Input: part model. Units: mm. Frame: model coordinates. A direction names the side the tool comes from. Round coordinates to 2 decimals unless told otherwise and drop trailing zeros. Loops run counter-clockwise (first coordinate to the right, second up) from the corner with the lowest first, then second, coordinate; pieces in that order, holes last. Notation, with made-up numbers: M 5,68.5 L 54,68.5 A9 cw 54,78.5 Z; hole C 29.5,20 d3. An arc over 180 degrees is marked long. Return JSON: item names as keys, results as strings. Group by question number.
1) Section A-A (y = 0). Output: boundary loops of the cut face in (x, z), plus the area to 3 significant figures.
2) Section C-C (x = 18). Output: boundary loops of the cut face in (y, z), plus the area to 3 significant figures.
3) Section B-B (z = 1.75). Output: boundary loops of the cut face in (x, y), plus the area to 3 significant figures.
4) Section D-D (x = -32). Output: boundary loops of the cut face in (y, z), plus the area to 3 significant figures.
5) Material intervals for line 1 (Z direction, x = -37, y = -14.5); line 2 (Y direction, x = -8, z = 7.25); line 3 (X direction, y = -2.5, z = 22.75), sorted ascending. Write a range as from..to.
6) Contact query for flat-ended pins moving along their axis: P1, Ø5, axis at x = -15, y = -11, coming from the +Z side; P2, Ø10, axis at x = -31.5, z = 13, coming from the -Y side; P3, Ø8.5, axis at x = -24, z = 7, coming from the +Y side. Output: stop coordinate, or through.
7) Access query for faces 4 (the face through (-28, 16.883, 5)), 5 (the face through (-29, 4, 10.668)), 6 (the face through (-20, -2.902, 13)). Directions: +Z, -Z, +X, -X, +Y, -Y. A direction counts if a zero-diameter tool reaches every point of the face in a straight line with its end or side. Return the directions, or none.
8) Mould query, pull axis Y, two halves, no side actions, for faces 1 (the face through (-55.367, 0, 5)), 2 (the face through (8.39, -9.46, 12.52)), 3 (the face through (-29, -16.883, 5)). Classes: +Y half, -Y half, draft (parallel to the pull), parting line (faces both ways), or undercut.
from build123d import *

# Parameters (mm, degrees)
F1_DEPTH = 10.668
F0_R     = 9.6911240881
F2_DEPTH = 25.4
F4_DEPTH = 9.144
F6_DEPTH = 23.4226514116


with BuildPart() as f1:
    # F0 (on Top) → F1 (new body)
    with BuildSketch(Plane.XY):
        with BuildLine():
            ThreePointArc((-1.1775513103, -16.8828442693), (-10.0338594761, 0), (-1.1775513103, 16.8828442693))
            Line((-1.1775513103, 16.8828442693), (-55.3673403338, 16.8828442693))
            Line((-55.3673403338, 16.8828442693), (-55.3673403338, -16.8828442693))
            Line((-55.3673403338, -16.8828442693), (-1.1775513103, -16.8828442693))
        make_face()
    extrude(amount=F1_DEPTH)

    # F0 (on Top) → F2 (join)
    with BuildSketch(Plane.XY):
        with BuildLine():
            ThreePointArc((31.0063367483, 0), (20.0186127494, 18.1716336717), (-1.1775513103, 16.8828442693))
            ThreePointArc((-1.1775513103, 16.8828442693), (-10.0338594761, 0), (-1.1775513103, -16.8828442693))
            ThreePointArc((-1.1775513103, -16.8828442693), (20.0186127494, -18.1716336717), (31.0063367483, 0))
        make_face()
        with Locations((10.4862386361, 0)):
            Circle(F0_R, mode=Mode.SUBTRACT)
    extrude(amount=F2_DEPTH)

    # F3 (on face) → F4 (join)
    with BuildSketch(Plane.XY.offset(10.668)):
        with BuildLine():
            ThreePointArc((-9.8276830676, -2.9015532994), (-10.0338594761, 0), (-9.8276830676, 2.9015532994))
            Line((-9.8276830676, 2.9015532994), (-46.7980072435, 2.9015532994))
            Line((-46.7980072435, 2.9015532994), (-46.7980072435, -2.9015532994))
            Line((-46.7980072435, -2.9015532994), (-9.8276830676, -2.9015532994))
        make_face()
    extrude(amount=F4_DEPTH)

    # F5 (on face) → F6 (cut, through all)
    with BuildSketch(Plane.XZ.offset(2.9015532994)):
        Polygon((-46.7980072435, 10.668), (-9.8276830676, 19.812), (-46.7980072435, 19.812), align=None)
    extrude(amount=-F6_DEPTH, mode=Mode.SUBTRACT)


solid = f1.part
Returned:
{
 "1": {"outline": "M -55.37,0 L 0.8,0 L 0.8,25.4 L -10.03,25.4 L -10.03,19.81 L -9.83,19.81 L -46.8,10.67 L -55.37,10.67 Z; M 20.18,0 L 31.01,0 L 31.01,25.4 L 20.18,25.4 Z", "area": "1,200 mm^2"},
 "2": {"outline": "M -19.09,0 L -6.12,0 L -6.12,25.4 L -19.09,25.4 Z; M 6.12,0 L 19.09,0 L 19.09,25.4 L 6.12,25.4 Z", "area": "659 mm^2"},
 "3": {"outline": "M -55.37,-16.88 L -1.18,-16.88 A20.52 ccw long -1.18,16.88 L -55.37,16.88 Z; hole C 10.49,0 d19.38", "area": "2,650 mm^2"},
 "4": {"outline": "M -16.88,0 L 16.88,0 L 16.88,10.67 L 2.9,10.67 L 2.9,14.33 L -2.9,14.33 L -2.9,10.67 L -16.88,10.67 Z", "area": "381 mm^2"},
 "5": {"line 1": "z = 0..10.67", "line 2": "y = -16.88..16.88", "line 3": "x = -9.88..1.12, 19.85..30.85"},
 "6": {"P1": "stops at z = 10.67", "P2": "stops at y = -16.88", "P3": "stops at y = 16.88"},
 "7": {"face 4": "+Z, -Z, -X, +Y", "face 5": "+Z, -X", "face 6": "+Z, -X, -Y"},
 "8": {"face 1": "draft", "face 2": "undercut", "face 3": "-Y half"}
}
